```python
from build123d import *

# Parameters (mm, degrees)
F0_R     = 11.079999938
F1_DEPTH = 7.04


with BuildPart() as f1:
    # F0 (on Front) → F1 (new body)
    with BuildSketch(Plane.XZ):
        with BuildLine():
            ThreePointArc((-28.8090031659, 22.2696470138), (-24.3900840083, 28.1937049584), (-22.8232076674, 35.4163227376))
            ThreePointArc((-22.8232076674, 35.4163227376), (-22.8405604112, 36.1938930103), (-22.8925840909, 36.9699150355))
            ThreePointArc((-22.8925840909, 36.9699150355), (-31.6310611427, 50.5643750287), (-47.7816925034, 51.1365903237))
            ThreePointArc((-47.7816925034, 51.1365903237), (-56.0085206864, 42.8711874283), (-57.1825180023, 31.2686309308))
            ThreePointArc((-57.1825180023, 31.2686309308), (-45.5226501495, 18.8019352041), (-28.8090031659, 22.2696470138))
        make_face()
        with Locations((-40.2532076054, 35.4163227376)):
            Circle(F0_R, mode=Mode.SUBTRACT)
        with BuildLine():
            ThreePointArc((-47.7816925034, 51.1365903237), (-31.6310611427, 50.5643750287), (-22.8925840909, 36.9699150355))
            Line((-22.8925840909, 36.9699150355), (-23.7404485644, 46.4443800767))
            ThreePointArc((-23.7404485644, 46.4443800767), (-23.2576465121, 49.4992381724), (-21.3890303605, 51.963691354))
            Line((-21.3890303605, 51.963691354), (-8.7265202555, 62.1209370132))
            ThreePointArc((-8.7265202555, 62.1209370132), (-25.2452652126, 61.0838938149), (-34.2931167989, 74.9432146938))
            Line((-34.2931167989, 74.9432146938), (-34.0369961774, 69.9059709762))
            ThreePointArc((-34.0369961774, 69.9059709762), (-35.2629924551, 62.1501768677), (-39.5130267128, 55.5477062744))
            ThreePointArc((-39.5130267128, 55.5477062744), (-40.3333403908, 54.8479164985), (-41.2602253247, 54.297004001))
            Line((-41.2602253247, 54.297004001), (-47.7816925034, 51.1365903237))
        make_face()
        with BuildLine():
            Line((-40.245373005, 12.314266868), (-28.8090031659, 22.2696470138))
            ThreePointArc((-28.8090031659, 22.2696470138), (-45.5226501495, 18.8019352041), (-57.1825180023, 31.2686309308))
            Line((-57.1825180023, 31.2686309308), (-57.0764976956, 27.7535374878))
            ThreePointArc((-57.0764976956, 27.7535374878), (-57.5592997479, 24.6986793921), (-59.4279158995, 22.2342262105))
            Line((-59.4279158995, 22.2342262105), (-68.3381404853, 15.0868802857))
            ThreePointArc((-68.3381404853, 15.0868802857), (-52.3672326621, 15.8542087629), (-42.4907709022, 3.2798621477))
            Line((-42.4907709022, 3.2798621477), (-42.5967912088, 6.7949555907))
            ThreePointArc((-42.5967912088, 6.7949555907), (-42.1139891566, 9.8498136864), (-40.245373005, 12.314266868))
        make_face()
        with BuildLine():
            Line((-6.5290846743, 63.8836122516), (-8.7265202555, 62.1209370132))
            ThreePointArc((-8.7265202555, 62.1209370132), (-7.5899744525, 62.955116416), (-6.5290846743, 63.8836122516))
        make_face()
        with BuildLine():
            ThreePointArc((-34.2931167989, 74.9432146938), (-25.2452652126, 61.0838938149), (-8.7265202555, 62.1209370132))
            Line((-8.7265202555, 62.1209370132), (-6.5290846743, 63.8836122516))
            ThreePointArc((-6.5290846743, 63.8836122516), (-2.7637901739, 69.3087740166), (-1.4373358773, 75.777958034))
            ThreePointArc((-1.4373358773, 75.777958034), (-18.2933365525, 92.2111495713), (-34.2931167989, 74.9432146938))
        make_face()
        with Locations((-17.8758302018, 75.777958034)):
            Circle(F0_R, mode=Mode.SUBTRACT)
        with BuildLine():
            ThreePointArc((-42.1793983078, 0), (-42.2574160625, 1.6473045105), (-42.4907709022, 3.2798621477))
            ThreePointArc((-42.4907709022, 3.2798621477), (-52.3672326621, 15.8542087629), (-68.3381404853, 15.0868802857))
            Line((-68.3381404853, 15.0868802857), (-72.4431903423, 11.7940102706))
            ThreePointArc((-72.4431903423, 11.7940102706), (-65.9383753509, -16.2403493387), (-42.1793983078, 0))
        make_face()
        with Locations((-59.6093982458, 0)):
            Circle(F0_R, mode=Mode.SUBTRACT)
        with BuildLine():
            Line((-72.4431903423, 11.7940102706), (-68.3381404853, 15.0868802857))
            ThreePointArc((-68.3381404853, 15.0868802857), (-70.5156565401, 13.5962652172), (-72.4431903423, 11.7940102706))
        make_face()
    extrude(amount=F1_DEPTH)


solid = f1.part
```
Can you work these out from the model? Positions are in its coordinate system, mm. A direction names the side the tool comes from. Give positions to 0.01 mm unless a question says otherwise; leave off trailing zeros. Write each loop counter-clockwise with the first axis right and the second up, starting at its lowest first coordinate (ties: lowest second). Pieces come first, ordered by that corner, then holes. Notation, with made-up numbers: (74, 38) -> (97, 38) arc R12 ccw to (97, 47) -> close; hole circle Ø8 at (-36.75, 39.25). An arc over 180 degrees is marked (long way). Write item = value, one per line.
(1) Suppose I cut it at D-D on z = 57.5. Write out the boundary of the cut face in (x, y).
Worked out:
outline = (-37.83, -7.04) -> (-14.49, -7.04) -> (-14.49, 0) -> (-37.83, 0) -> close
(2) Thinking about a two-plate mould opening in Z: for faces 1 (the face through (-63.82, -3.47, 18.71)), 2 (the face through (-34.61, -3.47, 17.22)), 3 (the face through (-31, -7.04, 42)), 4 (the face through (-57.54, -3.47, 24.74)), which applies, released by +Z, released by -Z, zero draft, split by the parting line, or undercut?
Worked out:
face_1 = released by +Z
face_2 = released by -Z
face_3 = zero draft
face_4 = undercut
(3) Suppose I cut it at A-A on x = -31. Write out the boundary of the cut face in (y, z).
Worked out:
outline = (-7.04, 20.36) -> (0, 20.36) -> (0, 29.32) -> (-7.04, 29.32) -> close; (-7.04, 41.51) -> (0, 41.51) -> (0, 85.68) -> (-7.04, 85.68) -> close
(4) I'm going to push flat-ended pins straight in: P1, Ø17.5, axis at x = -40.25, z = 35.42, coming from the +Y side; P2, Ø1, axis at x = -39.5, y = -3, coming from the +Z side; P3, Ø4, axis at y = -1.5, z = 7, coming from the +X side; P4, Ø1, axis at y = -1.5, z = 78.5, coming from the +X side. Where does each tip first touch, or does it pass through?
Worked out:
P1 = through
P2 = 56.09
P3 = -42.41
P4 = -1.59
(5) Suppose I cut it at B-B on z = 41.5. Write out the boundary of the cut face in (x, y).
Worked out:
outline = (-56.59, -7.04) -> (-49.51, -7.04) -> (-49.51, 0) -> (-56.59, 0) -> close; (-30.99, -7.04) -> (-23.3, -7.04) -> (-23.3, 0) -> (-30.99, 0) -> close
(6) For faces 5 (the face through (-35.224, -3.471, 62.254)), 6 (the face through (-23.31, -3.47, 41.64)), 7 (the face through (-34.3, -3.47, 44.76)), which set-ups out of +Z, -Z, +X, -X, +Y, -Y let a thin tool reach every point of the face, with its end or its side?
Worked out:
face_5 = -X, +Y, -Y
face_6 = +X, +Y, -Y
face_7 = +Y, -Y
(7) I need wall thicknesses on probe 1 along X at (y, z) = (-4.5, 44.5); probe 2 along X at (y, z) = (-2.5, 9); probe 3 along Z at (x, y) = (-27, -2). Which ranges of each line are inside material? Lowest first, please. Write a range as from..to.
Worked out:
probe_1 = -55.13..-46.6, -33.91..-23.57
probe_2 = -74.54..-66.07, -53.15..-42.41
probe_3 = 24.1..69.49, 82.06..89.45
(8) Suppose I cut it at C-C on y = -2.25. Write out the boundary of the cut face in (x, z), then the cut area to 3 significant figures.
Worked out:
outline = (-68.34, 15.09) arc R17.43 ccw (long way) to (-42.49, 3.28) -> (-42.6, 6.79) arc R6.35 cw to (-40.25, 12.31) -> (-28.81, 22.27) arc R17.43 ccw to (-22.89, 36.97) -> (-23.74, 46.44) arc R6.35 cw to (-21.39, 51.96) -> (-8.73, 62.12) arc R16.44 ccw (long way) to (-34.29, 74.94) -> (-34.04, 69.91) arc R19.05 cw to (-39.51, 55.55) arc R6.35 cw to (-41.26, 54.3) -> (-47.78, 51.14) arc R17.43 ccw to (-57.18, 31.27) -> (-57.08, 27.75) arc R6.35 cw to (-59.43, 22.23) -> close; hole circle Ø22.16 at (-59.61, 0); hole circle Ø22.16 at (-40.25, 35.42); hole circle Ø22.16 at (-17.88, 75.78)
area = 2,080 mm^2
